Read the model definition and answer for the solid it produces. Units are mm, in the model's axes. A direction names the side the tool comes from. Give positions to 0.01 mm unless a question says otherwise; leave off trailing zeros. Order: outer loops, then holes, each group sorted by start corner. A loop starts at its lowest first (then second) coordinate and runs counter-clockwise, first axis right, second up. Notation, with made-up numbers: (83.25, -27) - (110.25, -27) arc R13 cw to (110.25, -10) - close; hole circle Ø8 at (-6, -7). An arc over 180 degrees is marked (long way). Write item = value, one per line.
Autodesk Inventor part; units mm, degrees
ref_plane "Płaszczyzna konstrukcyjna2" through (-6, 5, 0) normal (0, 0, 1) x (1, 0, 0)
ref_plane "YZ Plane" through (0, 0, 0) normal (1, 0, 0) x (0, 1, 0)
ref_plane "XZ Plane" through (0, 0, 0) normal (0, 1, 0) x (-1, 0, 0)
sketch "Szkic3" plane through (0, 0, 0) normal (0, 1, 0) x (-1, 0, 0)
  circle A0 centre (0, 0) radius 5
  line L0 (-6, -6) -> (6, -6)
  line L1 (6, -6) -> (6, 6)
  line L2 (6, 6) -> (-6, 6)
  line L3 (-6, 6) -> (-6, -6)
  line L4 (-6, -6) -> (6, 6) construction
  line L5 (6, -6) -> (-6, 6) construction
  dimension "d12" = 10
  dimension "d15" = 12
  dimension "d16" = 12
extrude "Wyciągnięcie proste3" add sketch "Szkic3" along normal mid plane 10
extrude "Wyciągnięcie proste4" add sketch "Szkic3" along normal blind 5 contours A0
ref_plane "Płaszczyzna konstrukcyjna2" through (-6, 5, 0) normal (0, 0, 1) x (1, 0, 0)
sketch "Szkic7" plane through (-6, 5, 0) normal (0, 0, 1) x (1, 0, 0)
  line L0 (0, 0) -> (12, 0)
  line L1 (0, 0) -> (12, 0)
  line L2 (6, 0) -> (6, 6)
  line L3 (6, 0) -> (12, 0) construction
  circle A0 centre (6, 6) radius 2
  line L4 (4.2679, 5) -> (3.2679, 5)
  line L5 (6, 8) -> (6, 9)
  line L6 (7.7321, 5) -> (8.7321, 5)
  arc A1 (0, 0) -> (3.2679, 5) centre (-2.722, 5.347) ccw
  arc A2 (6, 9) -> (3.2679, 5) centre (6.0958, 6.0015) ccw
  arc A3 (8.7321, 5) -> (6, 9) centre (5.9042, 6.0015) ccw
  arc A4 (8.7321, 5) -> (12, 0) centre (14.722, 5.347) ccw
  point P0 (6, -5)
  dimension "d42" = 6
  dimension "d43" = 90
  dimension "d44" = 4
  dimension "d45" = 1
  dimension "d46" = 1
  dimension "d47" = 1
  dimension "d48" = 5
  dimension "d49" = 5
  dimension "d50" = 0
  dimension "d51" = 6
  dimension "d52" = 3
  dimension "d53" = 3
  dimension "d54" = 6
extrude "Wyciągnięcie proste7" add sketch "Szkic7" along normal mid plane 12 contours A1 L4 A0 L2 L0 | L2 A0 L6 A4 L0 | A2 L5 A0 L4 | A3 L6 A0 L5
sketch "Szkic8" plane through (-6, 5, 0) normal (0, 0, 1) x (1, 0, 0)
  arc A0 (8.7321, 5) -> (12, 0) centre (14.722, 5.347) ccw
  line L0 (0, 12) -> (12, 12)
  line L1 (12, 12) -> (12, 0)
  line L2 (12, 0) -> (0, 0)
  line L3 (0, 0) -> (0, 12)
  circle A1 centre (6, 6) radius 2
  line L4 (0, 12) -> (12, 0) construction
  line L5 (12, 12) -> (0, 0) construction
  point P0 (6, -5)
extrude "Wyciągnięcie proste8" cut sketch "Szkic8" along normal mid plane 4
fillet "Zaokrąglenie5" radius 6 2 edges at (6, 5, 0) (-6, 5, 0)
fillet "Zaokrąglenie6" radius 4 4 edges at (6, 0, 6) (6, 0, -6) (-6, 0, -6) (-6, 0, 6)
properties part number "Connector_hollow"
1. Section B-B (y = -2.75) is taken. Determine the outline of the cut face in (x, z), and give its area (3 significant figures).
Recorded:
outline = (-6, -2) arc R4 ccw to (-2, -6) - (2, -6) arc R4 ccw to (6, -2) - (6, 2) arc R4 ccw to (2, 6) - (-2, 6) arc R4 ccw to (-6, 2) - close; hole circle Ø10 at (0, 0)
area = 51.7 mm^2
2. Straight lines are drawn through the part: L1, parallel to X at y = 11, z = 4.7; L2, parallel to Z at x = 2.75, y = 6.5; L3, parallel to Z at x = 2, y = 9.75. For each, find the intervals that lie inside material, in ascending order. Write a range as [from, to].
Recorded:
L1 = [-2.9, -2], [2, 2.9]
L2 = [-5.93, -2], [2, 5.93]
L3 = [-6, -2], [2, 6]
3. Determine the mould class of faces 1 (the face through (-6, -3, 0)), 2 (the face through (0, 7, -2)), 3 (the face through (0, 13, -4)), 4 (the face through (6, -3, 0)) for opening direction X: +X half, -X half, draft (parallel to the pull), parting line (faces both ways), or undercut.
Recorded:
face_1 = -X half
face_2 = draft
face_3 = undercut
face_4 = +X half
4. Flat-ended cylindrical pins translate along their axes: pin 1 (2 mm diameter, centred on x = 4, z = -2, fed in from -Y); pin 2 (1 mm diameter, centred on x = 2.5, z = -0.5, fed in from +Y); pin 3 (3 mm diameter, centred on x = -3, z = -2.5, fed in from +Y); pin 4 (3 mm diameter, centred on y = 9.5, z = -4, fed in from +X). Find the tip coordinate at first contact, or state that the pin passes through.
Recorded:
pin_1 = -5
pin_2 = 4.66
pin_3 = 13.54
pin_4 = 3.2
5. Section D-D (x = 2.25) is taken. Determine the outline of the cut face in (y, z).
Recorded:
outline = (-5, -5.99) - (12.87, -5.99) - (12.87, -2) - (4.56, -2) - (4.56, 2) - (12.87, 2) - (12.87, 5.99) - (-5, 5.99) - (-5, 4.47) - (0, 4.47) - (0, -4.47) - (-5, -4.47) - close
6. For faces 5 (the face through (4.859, 2.184, -4.797)), 6 (the face through (-4.196, 3.289, 0.028)), 7 (the face through (-3.676, 7.101, 3.939)), 8 (the face through (3.374, 7.628, 3.939)), determine the directions among +Z, -Z, +X, -X, +Y, -Y from which every point of the face is accessible in a straight line to the end or side of a thin tool.
Recorded:
face_5 = -Z, +X, +Y, -Y
face_6 = -X, +Y
face_7 = +Z, -Z, -X
face_8 = +Z, -Z, +X
7. Section A-A (y = 11.25) is taken. Count the separate pieces of the cut face and the enclosed holes in it, and give its area (3 significant figures).
Recorded:
separate_pieces = 4
enclosed_holes = 0
area = 14.4 mm^2
